Autodesk Inventor part; units mm, degrees
ref_plane "YZ Plane" through (0, 0, 0) normal (1, 0, 0) x (0, 1, 0)
ref_plane "XZ Plane" through (0, 0, 0) normal (0, 1, 0) x (-1, 0, 0)
ref_plane "XY Plane" through (0, 0, 0) normal (0, 0, 1) x (1, 0, 0)
sketch "Sketch1" plane through (0, 0, 0) normal (0, 1, 0) x (-1, 0, 0)
  line L0 (33.1574, 54.0426) -> (-23.9926, 54.0426)
  line L1 (-23.9926, 54.0426) -> (-23.9926, -57.0824)
  line L2 (-23.9926, -57.0824) -> (33.1574, -57.0824)
  line L3 (33.1574, -57.0824) -> (33.1574, 54.0426)
  point P0 (0, 0)
  dimension "d0" = 111.125
  dimension "d1" = 57.15
extrude "Extrusion1" add sketch "Sketch1" along normal blind 1.5875
sketch "Sketch2" plane through (0, 1.5875, 0) normal (0, 1, 0) x (1, 0, 0)
  line L0 (-31.5699, -52.4551) -> (22.4051, -52.4551)
  line L1 (22.4051, -52.4551) -> (22.4051, 55.4949)
  line L2 (22.4051, 55.4949) -> (-31.5699, 55.4949)
  line L3 (-31.5699, 55.4949) -> (-31.5699, -52.4551)
  line L4 (-33.1574, -54.0426) -> (23.9926, -54.0426)
  line L5 (23.9926, -54.0426) -> (23.9926, 57.0824)
  line L6 (23.9926, 57.0824) -> (-33.1574, 57.0824)
  line L7 (-33.1574, 57.0824) -> (-33.1574, -54.0426)
  point P0 (0, 0)
  dimension "d4" = 1.5875
  dimension "d5" = 1.5875
  dimension "d6" = 1.5875
  dimension "d7" = 1.5875
extrude "Extrusion2" add sketch "Sketch2" along normal blind 1.5875 contours L3 L2 L1 L0
properties part number "SD_BaseStation_Lid"
Design review of the part built by this model. Coordinates are the model's own, in mm. Coordinates: 2 decimals unless noted, no trailing zeros. Order: outer loops, then holes, each group sorted by start corner. A loop starts at its lowest first (then second) coordinate and runs counter-clockwise, first axis right, second up.
1) Wall thickness on line 1 along Z through (x, y) = (-15.5, 1.8); line 2 along X through (y, z) = (3, 26): over which ranges is each line inside the solid? List them lowest first.
2) Clearance check with flat-ended pins moving along their axes: pin 1 (0.5 mm diameter, centred on x = -9, y = 2, fed in from +Z); pin 2 (1.7 mm diameter, centred on y = 2.5, z = 2, fed in from -X); pin 3 (0.5 mm diameter, centred on x = -13.5, y = 2, fed in from -Z). State where each tip first meets the part, or that it passes through.
3) Take a section at A-A, the plane z = 10. Give the boundary of the cut face in (x, y) (1 decimal), and give its area (3 significant figures).
4) Take a section at B-B, the plane y = 2.2. Give the boundary of the cut face in (x, z), and give its area (3 significant figures).
Returned:
1. line 1: z = -55.49 to 52.46
1. line 2: x = -31.57 to 22.41
2. pin 1: stops at z = 52.46
2. pin 2: stops at x = -31.57
2. pin 3: stops at z = -55.49
3. outline: (-33.2, 0) - (24, 0) - (24, 1.6) - (22.4, 1.6) - (22.4, 3.2) - (-31.6, 3.2) - (-31.6, 1.6) - (-33.2, 1.6) - close
3. area: 176 mm2
4. outline: (-31.57, -55.49) - (22.41, -55.49) - (22.41, 52.46) - (-31.57, 52.46) - close
4. area: 5,830 mm2
